The model under review builds one solid part; all positions refer to its coordinate system, in mm. Face numbers are marked on the shaded views. A direction names the side the tool comes from. Coordinates: 2 decimals unless noted, no trailing zeros. Write each loop counter-clockwise with the first axis right and the second up, starting at its lowest first coordinate (ties: lowest second). Pieces come first, ordered by that corner, then holes. Notation, with made-up numbers: (40, 24) - (62, 24) arc R9 ccw to (62, 40) - close; hole circle Ø9 at (16, 9.25). An arc over 180 degrees is marked (long way). Put each result on its own line as item: value.
from build123d import *

# Parameters (mm, degrees)
SKETCH1_W           = 9.5
SKETCH1_H           = 11
BOSS_EXTRUDE1_DEPTH = 3
SKETCH2_R           = 4.3
CUT_EXTRUDE1_DEPTH  = 2
FILLET1_R           = 2
SKETCH3_W           = 9.5
SKETCH3_H           = 4
CUT_EXTRUDE2_DEPTH  = 2
SKETCH4_W           = 0.6
SKETCH4_H           = 3
BOSS_EXTRUDE2_DEPTH = 3.7
SKETCH5_W           = 0.5
SKETCH5_H           = 1.2
BOSS_EXTRUDE3_DEPTH = 3
CUT_EXTRUDE3_DEPTH  = 10.932396488
SKETCH7_R           = 0.5
BOSS_EXTRUDE4_DEPTH = 1
FILLET2_R           = 0.2
SKETCH8_R           = 4
SKETCH8_W           = 1
SKETCH8_H           = 2
BOSS_EXTRUDE5_DEPTH = 2


with BuildPart() as part:
    # Sketch1 → Boss-Extrude1 (new body)
    with BuildSketch(Plane.XY):
        Rectangle(SKETCH1_W, SKETCH1_H)
    extrude(amount=BOSS_EXTRUDE1_DEPTH)

    # Sketch2 → Cut-Extrude1 (cut)
    with BuildSketch(Plane.XY.offset(3)):
        with Locations((0, 0.6)):
            Circle(SKETCH2_R)
    extrude(amount=-CUT_EXTRUDE1_DEPTH, mode=Mode.SUBTRACT)

    # Fillet1
    fillet1_edges = [part.edges().sort_by_distance(p)[0] for p in [
        (-4.75, 5.5, 1.5),
        (4.75, 5.5, 1.5),
    ]]
    fillet(fillet1_edges, radius=FILLET1_R)

    # Sketch3 → Cut-Extrude2 (cut)
    with BuildSketch(Plane.XY.offset(3)):
        Rectangle(SKETCH3_W, SKETCH3_H)
    extrude(amount=-CUT_EXTRUDE2_DEPTH, mode=Mode.SUBTRACT)

    # Sketch4 → Boss-Extrude2 (add)
    with BuildSketch(Plane.XY.offset(1)):
        with Locations((-4.45, 0)):
            Rectangle(SKETCH4_W, SKETCH4_H)
        with Locations((4.45, 0)):
            Rectangle(SKETCH4_W, SKETCH4_H)
    extrude(amount=BOSS_EXTRUDE2_DEPTH)

    # Sketch5 → Boss-Extrude3 (add)
    with BuildSketch(Plane.XZ.offset(1.5)):
        with Locations((5, 4.1)):
            Rectangle(SKETCH5_W, SKETCH5_H)
        with Locations((-5, 4.1)):
            Rectangle(SKETCH5_W, SKETCH5_H)
    extrude(amount=-BOSS_EXTRUDE3_DEPTH)

    # Sketch6 → Cut-Extrude3 (cut, through all)
    with BuildSketch(Plane.XZ.offset(1.5)):
        Polygon((5.25, 3.5), (4.25, 4.7), (5.25, 4.7), align=None)
        Polygon((-5.25, 3.5), (-4.25, 4.7), (-5.25, 4.7), align=None)
    extrude(amount=-CUT_EXTRUDE3_DEPTH, mode=Mode.SUBTRACT)

    # Sketch7 → Boss-Extrude4 (add)
    with BuildSketch(Plane.XY.offset(3)):
        with Locations(Location((-3.75, 4, 0), (0, 0, 180))):
            Circle(SKETCH7_R)
        with Locations(Location((3.75, 4, 0), (0, 0, 180))):
            Circle(SKETCH7_R)
        with Locations(Location((-3.75, -4.5, 0), (0, 0, 180))):
            Circle(SKETCH7_R)
    extrude(amount=BOSS_EXTRUDE4_DEPTH)

    # Fillet2
    fillet2_edges = [part.edges().sort_by_distance(p)[0] for p in [
        (-3.25, 4, 4),
        (4.25, 4, 4),
        (-3.25, -4.5, 4),
    ]]
    fillet(fillet2_edges, radius=FILLET2_R)

    # Sketch8 → Boss-Extrude5 (add)
    with BuildSketch(Plane.XY.offset(1)):
        with Locations(Location((0, 0.6, 0), (0, 0, 180))):
            Circle(SKETCH8_R)
        with Locations((0, 0.6)):
            Rectangle(SKETCH8_W, SKETCH8_H, mode=Mode.SUBTRACT)
    extrude(amount=BOSS_EXTRUDE5_DEPTH)


solid = part.part
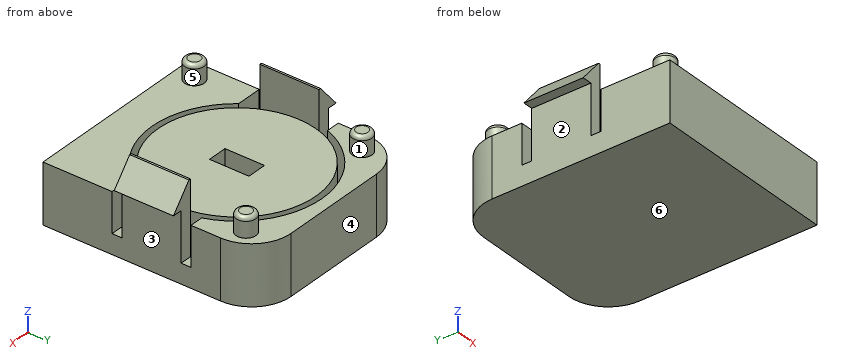
1. Consider section D-D on x = -3.75. State the section outline as (y, z) points.
Determined:
outline: (-5.5, 0) - (5.23, 0) - (5.23, 3) - (4.5, 3) - (4.5, 3.8) arc R0.2 ccw to (4.3, 4) - (3.7, 4) arc R0.2 ccw to (3.5, 3.8) - (3.5, 3) - (2.7, 3) - (2.7, 1) - (1.99, 1) - (1.99, 3) - (-0.79, 3) - (-0.79, 1) - (-2, 1) - (-2, 3) - (-4, 3) - (-4, 3.8) arc R0.2 ccw to (-4.2, 4) - (-4.8, 4) arc R0.2 ccw to (-5, 3.8) - (-5, 3) - (-5.5, 3) - close
2. Consider section A-A on x = 0. State the section outline as (y, z) points.
Determined:
outline: (-5.5, 0) - (5.5, 0) - (5.5, 3) - (4.9, 3) - (4.9, 1) - (4.6, 1) - (4.6, 3) - (1.6, 3) - (1.6, 1) - (-0.4, 1) - (-0.4, 3) - (-3.4, 3) - (-3.4, 1) - (-3.7, 1) - (-3.7, 3) - (-5.5, 3) - close
3. Machinability: for the marked faces 1, 2 and 3, which of the approach directions +Z, -Z, +X, -X, +Y, -Y give a long, thin tool a straight path to every point of the face, cutting with its end or side? Answer none if there is none.
Determined:
face 1: +Z
face 2: -Z, -X, +Y, -Y
face 3: -Z, +X, +Y, -Y
4. Consider section C-C on y = -3.25. State the section outline as (x, z) points, plus the area to 3 significant figures.
Determined:
outline: (-4.75, 0) - (4.75, 0) - (4.75, 3) - (1.92, 3) - (1.92, 1) - (1.09, 1) - (1.09, 3) - (-1.09, 3) - (-1.09, 1) - (-1.92, 1) - (-1.92, 3) - (-4.75, 3) - close
area: 25.2 mm^2
5. To check wall thickness, follow probe 1 along X at (y, z) = (-0.25, 3.1); probe 2 along X at (y, z) = (3, 1.65); probe 3 along X at (y, z) = (4, 1.1). State the ranges of each line that lie inside material, in increasing order.
Determined:
probe 1: x = -4.75 to -4.15, 4.15 to 4.75
probe 2: x = -4.75 to -3.57, -3.2 to 3.2, 3.57 to 4.75
probe 3: x = -4.69 to -2.63, -2.11 to 2.11, 2.63 to 4.69
6. Consider section B-B on y = -4.5. State the section outline as (x, z) points, plus the area to 3 significant figures.
Determined:
outline: (-4.75, 0) - (4.75, 0) - (4.75, 3) - (-3.25, 3) - (-3.25, 3.8) arc R0.2 ccw to (-3.45, 4) - (-4.05, 4) arc R0.2 ccw to (-4.25, 3.8) - (-4.25, 3) - (-4.75, 3) - close
area: 29.5 mm^2
7. The part is to be moulded in two halves that separate along Y. For the marked faces 4, 5 and 6, say which applies: +Y half, -Y half, draft (parallel to the pull), parting line (faces both ways), or undercut.
Determined:
face 4: +Y half
face 5: undercut
face 6: draft
8. For pin 1 Ø1.6 at (y, z) = (0.5, 2.5) entering from -X; pin 2 Ø0.7 at (x, z) = (-4.5, 2.5) entering from +Y; pin 3 Ø1.5 at (x, y) = (-2.5, -2) entering from +Z, all flat-tipped, find the tip position at first contact; note any pin that passes through.
Determined:
pin 1: stops at x = -4.75
pin 2: stops at y = 4.93
pin 3: stops at z = 3
